For this review, take the finished solid that the model builds, in its own axes (mm). Face numbers are marked on the shaded views. A direction names the side the tool comes from. Round coordinates to 2 decimals unless told otherwise and drop trailing zeros. Write each loop counter-clockwise with the first axis right and the second up, starting at its lowest first coordinate (ties: lowest second). Pieces come first, ordered by that corner, then holes. Notation, with made-up numbers: M 89,0.5 L 146,0.5 A24 cw 146,11.5 Z; hole C 50,25.25 d2. An arc over 180 degrees is marked long. One line per question, with ' | ' between items.
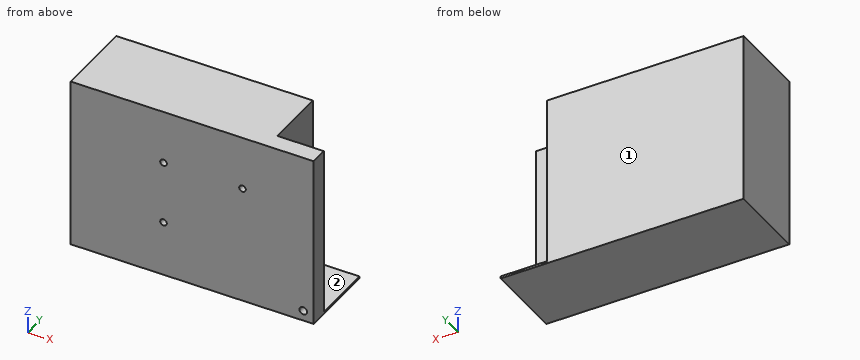
```python
from build123d import *

# Parameters (mm, degrees)
SKETCH1_W           = 110
SKETCH1_H           = 78
BOSS_EXTRUDE1_DEPTH = 36
SKETCH2_W           = 21.010174998
SKETCH2_H           = 77
CUT_EXTRUDE1_DEPTH  = 28
SKETCH3_R           = 1.725
CUT_EXTRUDE2_DEPTH  = 89.2743541
SKETCH4_R           = 1.5
CUT_EXTRUDE3_DEPTH  = 5


with BuildPart() as part:
    # Sketch1 → Boss-Extrude1 (new body)
    with BuildSketch(Plane(origin=(0, 0, 0), x_dir=(1, 0, 0), z_dir=(0, 1, 0))):
        with Locations((8.088235294, -16.029411765)):
            Rectangle(SKETCH1_W, SKETCH1_H)
    extrude(amount=BOSS_EXTRUDE1_DEPTH)

    # Sketch2 → Cut-Extrude1 (cut)
    with BuildSketch(Plane(origin=(0, 36, 0), x_dir=(1, 0, 0), z_dir=(0, 1, 0))):
        with Locations((52.583147795, -16.529411765)):
            Rectangle(SKETCH2_W, SKETCH2_H)
    extrude(amount=-CUT_EXTRUDE1_DEPTH, mode=Mode.SUBTRACT)

    # Sketch3 → Cut-Extrude2 (cut, through all)
    with BuildSketch(Plane(origin=(0, 8, 0), x_dir=(1, 0, 0), z_dir=(0, 1, 0))):
        with Locations(Location((58.363235294, 18.245588235, 0), (0, 0, 270))):
            Circle(SKETCH3_R)
    extrude(amount=-CUT_EXTRUDE2_DEPTH, mode=Mode.SUBTRACT)

    # Sketch4 → Cut-Extrude3 (cut)
    with BuildSketch(Plane.XZ):
        with Locations(Location((-4.911764706, 2.129411765, 0), (0, 0, 270))):
            Circle(SKETCH4_R)
        with Locations(Location((-4.911764706, 30.729411765, 0), (0, 0, 270))):
            Circle(SKETCH4_R)
        with Locations(Location((30.838235294, 30.729411765, 0), (0, 0, 270))):
            Circle(SKETCH4_R)
    extrude(amount=-CUT_EXTRUDE3_DEPTH, mode=Mode.SUBTRACT)


solid = part.part
```
Item 1: Take a section at B-B (y = 21). Write out the cut boundary in (x, z).
Results:
outline: M -46.91,-22.97 L 63.09,-22.97 L 63.09,-21.97 L 42.08,-21.97 L 42.08,55.03 L -46.91,55.03 Z
Item 2: To check wall thickness, follow line 1 along Y through (x, z) = (49, 35); line 2 along X through (y, z) = (27, 39). State the ranges of each line that lie inside material, in increasing order. Write a range as from..to.
Results:
line 1: 0..8 | line 2: -46.91..42.08
Item 3: Machinability: for the marked faces 1 and 2, which of the approach directions +Z, -Z, +X, -X, +Y, -Y give a long, thin tool a straight path to every point of the face, cutting with its end or side? Answer none if there is none.
Results:
face 1: +Z, -Z, +X, -X, +Y | face 2: +Z, +X, +Y
Item 4: Insertion check: pin 1 Ø3 at (y, z) = (15, 3) entering from +X; pin 2 Ø23 at (x, z) = (55.5, 9) entering from +Y; pin 3 Ø1.5 at (x, z) = (31, 31) entering from -Y. Each pin has a flat end and moves straight along its axis. Give the tip position at first contact, or say it passes through.
Results:
pin 1: x = 42.08 | pin 2: y = 8 | pin 3: y = 5
Item 5: Take a section at A-A (x = 54). Write out the cut boundary in (y, z).
Results:
outline: M 0,-22.97 L 36,-22.97 L 36,-21.97 L 8,-21.97 L 8,55.03 L 0,55.03 Z
